from build123d import *

# Parameters (mm, degrees)
BOSS_EXTRUDE1_DEPTH = 85
SKETCH3_R           = 10
SKETCH3_R_2         = 2.2
CUT_EXTRUDE1_DEPTH  = 85
SKETCH4_R           = 1.6
CUT_EXTRUDE2_DEPTH  = 85


with BuildPart() as part:
    # Sketch2 → Boss-Extrude1 (new body)
    with BuildSketch(Plane.XY):
        Polygon((0, 0), (87.594271247, 0), (83.452135624, 10), (4.142135624, 10), align=None)
    extrude(amount=BOSS_EXTRUDE1_DEPTH)

    # Sketch3 → Cut-Extrude1 (cut)
    with BuildSketch(Plane(origin=(0, 10, 0), x_dir=(1, 0, 0), z_dir=(0, 1, 0))):
        with Locations(Location((43.797135624, -42.734969619, 0), (0, 0, 180))):
            Circle(SKETCH3_R)
        with Locations(Location((43.797135624, -20.234969619, 0), (0, 0, 180))):
            Circle(SKETCH3_R_2)
        with Locations(Location((59.7070382, -26.825067042, 0), (0, 0, 180))):
            Circle(SKETCH3_R_2)
        with Locations(Location((66.297135624, -42.734969619, 0), (0, 0, 180))):
            Circle(SKETCH3_R_2)
        with Locations(Location((59.7070382, -58.644872196, 0), (0, 0, 180))):
            Circle(SKETCH3_R_2)
        with Locations(Location((43.797135624, -65.234969619, 0), (0, 0, 180))):
            Circle(SKETCH3_R_2)
        with Locations(Location((27.887233047, -58.644872196, 0), (0, 0, 180))):
            Circle(SKETCH3_R_2)
        with Locations(Location((21.297135624, -42.734969619, 0), (0, 0, 180))):
            Circle(SKETCH3_R_2)
        with Locations(Location((27.887233047, -26.825067042, 0), (0, 0, 180))):
            Circle(SKETCH3_R_2)
    extrude(amount=-CUT_EXTRUDE1_DEPTH, mode=Mode.SUBTRACT)

    # Sketch4 → Cut-Extrude2 (cut)
    with BuildSketch(Plane(origin=(0, 10, 0), x_dir=(1, 0, 0), z_dir=(0, 1, 0))):
        with Locations(Location((12.642135624, -20, 0), (0, 0, 180))):
            Circle(SKETCH4_R)
        with Locations(Location((12.642135624, -42.5, 0), (0, 0, 180))):
            Circle(SKETCH4_R)
        with Locations(Location((12.642135624, -65, 0), (0, 0, 180))):
            Circle(SKETCH4_R)
        with Locations(Location((74.952135624, -65, 0), (0, 0, 180))):
            Circle(SKETCH4_R)
        with Locations(Location((74.952135624, -42.5, 0), (0, 0, 180))):
            Circle(SKETCH4_R)
        with Locations(Location((74.952135624, -20, 0), (0, 0, 180))):
            Circle(SKETCH4_R)
    extrude(amount=-CUT_EXTRUDE2_DEPTH, mode=Mode.SUBTRACT)


solid = part.part
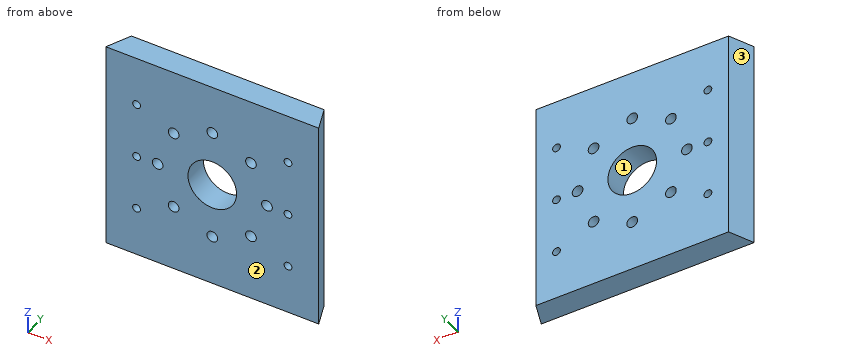
The listing builds one solid part. Answer for the finished solid, in the listing's coordinates (mm). Face numbers are marked on the shaded views. Give positions to 0.01 mm unless a question says otherwise; leave off trailing zeros. Write each loop counter-clockwise with the first axis right and the second up, starting at its lowest first coordinate (ties: lowest second). Pieces come first, ordered by that corner, then holes.
1) Given P1, Ø4, axis at y = 7.5, z = 35, coming from the +X side; P2, Ø1.5, axis at y = 1.5, z = 60.5, coming from the -X side, each flat-ended and moving along its own axis, determine where each tip first touches the part or whether it passes through.
2) Section B-B (y = 3.75) is taken. Count the separate pieces of the cut face and the enclosed holes in it, and give its area (3 significant figures).
3) Section C-C (x = 59) is taken. Write down the section's boundary in (y, z).
4) For a pull along X with two mould halves and no side action, classify the marked faces 1, 2 and 3 as pulls with the +X half, pulls with the -X half, needs draft (parallel to the pull), parting line crosses it, or undercut.
5) Find the intervals of material crossed by L1, parallel to Z at x = 61.5, y = 8.25; L2, parallel to Z at x = 42, y = 9.25; L3, parallel to X at y = 8, z = 64, in increasing order.
6) Section A-A (z = 47.5) is taken. Write down the section's boundary in (x, y).
Response:
1. P1: stops at x = 85.32
1. P2: stops at x = 0.31
2. separate pieces: 1
2. enclosed holes: 15
2. area: 6,700 mm2
3. outline: (0, 0) - (10, 0) - (10, 24.74) - (0, 24.74) - close; (0, 28.91) - (10, 28.91) - (10, 56.56) - (0, 56.56) - close; (0, 60.73) - (10, 60.73) - (10, 85) - (0, 85) - close
4. face 1: undercut
4. face 2: needs draft
4. face 3: pulls with the -X half
5. L1: z = 0 to 25.55, 28.1 to 57.37, 59.92 to 85
5. L2: z = 0 to 18.97, 21.5 to 32.9, 52.57 to 63.97, 66.5 to 85
5. L3: x = 3.31 to 11.39, 13.89 to 41.98, 45.62 to 73.7, 76.2 to 84.28
6. outline: (0, 0) - (35.01, 0) - (35.01, 10) - (4.14, 10) - close; (52.59, 0) - (87.59, 0) - (83.45, 10) - (52.59, 10) - close
